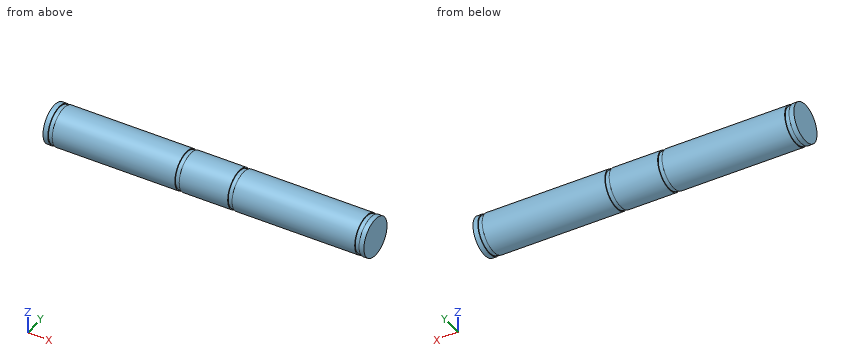
```python
from build123d import *


with BuildPart() as part:
    # Sketch1 → Revolve1 (revolve)
    with BuildSketch(Plane.XY, mode=Mode.PRIVATE) as revolve1_sk:
        Polygon((0, 0), (64.3, 0), (64.3, 4), (63.3, 4), (63.3, 3.8), (62.4, 3.8), (62.4, 4), (37.1, 4), (37.1, 3.8), (36.2, 3.8), (36.2, 4), (26.2, 4), (26.2, 3.8), (25.3, 3.8), (25.3, 4), (0, 4), (0, 3.8), (-0.9, 3.8), (-0.9, 4), (-1.9, 4), (-1.9, 0), align=None)
    revolve(revolve1_sk.sketch.rotate(Axis((0, 0, 0), (1, 0, 0)), 180), axis=Axis((0, 0, 0), (1, 0, 0)))


solid = part.part
```
For this review, take the finished solid that the model builds, in its own axes (mm). Coordinates: 2 decimals unless noted, no trailing zeros. Order: outer loops, then holes, each group sorted by start corner. A loop starts at its lowest first (then second) coordinate and runs counter-clockwise, first axis right, second up. Notation, with made-up numbers: (-38, -29.75) -> (-33, -29.75) arc R26 ccw to (-33, 9.25) -> close; hole circle Ø2 at (-14.75, -8). An arc over 180 degrees is marked (long way). Answer as CSV lines item,"result".
Q1. Clearance check with flat-ended pins moving along their axes: pin 1 Ø3 at (x, y) = (38, 2) entering from +Z; pin 2 Ø1.5 at (x, y) = (39.5, 2) entering from +Z. State where each tip first meets the part, or that it passes through.
Model answer:
pin 1,"stops at z = 3.97"
pin 2,"stops at z = 3.8"
Q2. We need section A-A (x = 31). State the section outline as (y, z) points.
Model answer:
outline,"circle Ø8 at (0, 0)"
Q3. Wall thickness on line 1 along Z through (x, y) = (1, 0.25); line 2 along Y through (x, z) = (57, 3.25); line 3 along Z through (x, y) = (44, -2): over which ranges is each line inside the solid? List them lowest first. Write a range as [from, to].
Model answer:
line 1,"z = [-3.99, 3.99]"
line 2,"y = [-2.33, 2.33]"
line 3,"z = [-3.46, 3.46]"
